from build123d import *

# Parameters (mm, degrees)
BOSS_EXTRU_1_DEPTH                                = 53.6
BOSS_EXTRU_1_DEPTH_BACK                           = 0.0001
ESQUISSE1_W                                       = 102.6
ESQUISSE1_H                                       = 35
ESQUISSE4_W                                       = 98.6
ESQUISSE4_H                                       = 51.6
ENL_V_MAT_EXTRU_2_DEPTH                           = 33
ESQUISSE9_W                                       = 10
ESQUISSE9_H                                       = 12.38
BOSS_EXTRU_3_DEPTH                                = 21.5
CONG_1_R                                          = 5
ESQUISSE10_R                                      = 3.75
ENL_V_MAT_EXTRU_4_DEPTH                           = 15
ENL_V_MAT_EXTRU_5_DEPTH                           = 2.1
ESQUISSE19_W                                      = 102.6
ESQUISSE19_H                                      = 53.6001
BOSS_EXTRU_4_DEPTH                                = 5
ESQUISSE21_W                                      = 5
ESQUISSE21_H                                      = 40
BOSS_EXTRU_5_DEPTH                                = 12
ESQUISSE22_W                                      = 5
ESQUISSE22_H                                      = 40
BOSS_EXTRU_6_DEPTH                                = 12
FRAISAGE_POUR_VIS_T_TE_FRAIS_E_BOMB_E_D           = 5.09999996
FRAISAGE_POUR_VIS_T_TE_FRAIS_E_BOMB_E_CSINK_D     = 10.500000082
FRAISAGE_POUR_VIS_T_TE_FRAIS_E_BOMB_E_CSINK_ANGLE = 90


with BuildPart() as part:
    # Esquisse1 → Boss.-Extru.1 (new, two sides: drawn at the far end of the back side and taken through both)
    with BuildSketch(Plane.XY.offset(-BOSS_EXTRU_1_DEPTH_BACK)):
        with Locations((33.832170394, 1.686746988)):
            Rectangle(ESQUISSE1_W, ESQUISSE1_H)
    extrude(amount=BOSS_EXTRU_1_DEPTH + BOSS_EXTRU_1_DEPTH_BACK)

    # Esquisse4 → Enlèv. mat.-Extru.2 (cut)
    with BuildSketch(Plane(origin=(0, 19.186746988, 0), x_dir=(1, 0, 0), z_dir=(0, 1, 0))):
        with Locations((33.832170394, -25.7999)):
            Rectangle(ESQUISSE4_W, ESQUISSE4_H)
    extrude(amount=-ENL_V_MAT_EXTRU_2_DEPTH, mode=Mode.SUBTRACT)

    # Esquisse9 → Boss.-Extru.3 (add)
    with BuildSketch(Plane(origin=(0, -13.813253012, 0), x_dir=(1, 0, 0), z_dir=(0, 1, 0))):
        with Locations((1.532170394, -32.0399)):
            Rectangle(ESQUISSE9_W, ESQUISSE9_H)
        with Locations((66.132170394, -32.0399)):
            Rectangle(ESQUISSE9_W, ESQUISSE9_H)
    extrude(amount=BOSS_EXTRU_3_DEPTH)

    # Congé1
    cong_1_edges = [part.edges().sort_by_distance(p)[0] for p in [
        (-3.467829606, 7.686746988, 32.0399),
        (6.532170394, 7.686746988, 32.0399),
        (71.132170394, 7.686746988, 32.0399),
        (61.132170394, 7.686746988, 32.0399),
    ]]
    fillet(cong_1_edges, radius=CONG_1_R - 0.0001)  # a hair under: the kernel refuses the full size

    # Esquisse10 → Enlèv. mat.-Extru.4 (cut)
    with BuildSketch(Plane(origin=(0, 0, 25.8499), x_dir=(-1, 0, 0), z_dir=(0, 0, -1))):
        with Locations((-66.132170394, 2.186746988)):
            Circle(ESQUISSE10_R)
        with Locations((-1.532170394, 2.186746988)):
            Circle(ESQUISSE10_R)
    extrude(amount=-ENL_V_MAT_EXTRU_4_DEPTH, mode=Mode.SUBTRACT)

    # Esquisse18 → Enlèv. mat.-Extru.5 (cut)
    with BuildSketch(Plane.XY.offset(53.6)):
        with BuildLine():
            Line((24.333519225, -13.813253012), (44.330821563, -13.813253012))
            ThreePointArc((44.330821563, -13.813253012), (34.332170394, -3.643205178), (24.333519225, -13.813253012))
        make_face()
    extrude(amount=-ENL_V_MAT_EXTRU_5_DEPTH, mode=Mode.SUBTRACT)

    # Esquisse19 → Boss.-Extru.4 (add)
    with BuildSketch(Plane.XZ.offset(15.813253012)):
        with Locations((33.832170394, 26.79995)):
            Rectangle(ESQUISSE19_W, ESQUISSE19_H)
    extrude(amount=BOSS_EXTRU_4_DEPTH)

    # Esquisse21 → Boss.-Extru.5 (add)
    with BuildSketch(Plane.ZY.offset(17.467829606)):
        with Locations((2.4999, -0.813253012)):
            Rectangle(ESQUISSE21_W, ESQUISSE21_H)
    extrude(amount=BOSS_EXTRU_5_DEPTH)

    # Esquisse22 → Boss.-Extru.6 (add)
    with BuildSketch(Plane(origin=(85.132170394, 0, 0), x_dir=(0, 0, -1), z_dir=(1, 0, 0))):
        with Locations((-2.4999, -0.813253012)):
            Rectangle(ESQUISSE22_W, ESQUISSE22_H)
    extrude(amount=BOSS_EXTRU_6_DEPTH)

    # Fraisage pour vis à tête fraisée bombée #51 (through all)
    with Locations(Plane(origin=(91.132170394, 13.186746988, -0.0001), x_dir=(-1, 0, 0), z_dir=(0, 0, -1))):
        with Locations((0, 0), (0, -28), (114.6, 0), (114.6, -28)):
            CounterSinkHole(FRAISAGE_POUR_VIS_T_TE_FRAIS_E_BOMB_E_D / 2, FRAISAGE_POUR_VIS_T_TE_FRAIS_E_BOMB_E_CSINK_D / 2, counter_sink_angle=FRAISAGE_POUR_VIS_T_TE_FRAIS_E_BOMB_E_CSINK_ANGLE)


solid = part.part
For this review, take the finished solid that the model builds, in its own axes (mm). A direction names the side the tool comes from. Give positions to 0.01 mm unless a question says otherwise; leave off trailing zeros. Loops run counter-clockwise (first coordinate to the right, second up) from the corner with the lowest first, then second, coordinate; pieces in that order, holes last. Notation, with made-up numbers: M 31,42.5 L 71,42.5 A32 cw 71,76.5 Z; hole C 30,32.5 d2. An arc over 180 degrees is marked long. Answer as a JSON object with one key per item and string values. Group by question number.
Q1. Add section B-B on x = 41. Give the boundary of the cut face in (y, z), and give its area (3 significant figures).
Q2. Mouldability with a two-part tool opening along Y and no side actions: class faces 1 (the conical face through (-20.91, 13.99, 2.57)), 2 (the flat face through (34, -14, 0)), 3 (the cylindrical face through (69.71, 6.18, 31.95)) as +Y half, -Y half, draft (parallel to the pull), parting line (faces both ways), or undercut.
Q3. For probe 1 along X at (y, z) = (1, 45.5); probe 2 along X at (y, z) = (-9, 28); probe 3 along X at (y, z) = (0, 27), list the stretches that pass through material, from the lowest coordinate up. Write a range as [from, to].
Q4. Add section A-A on z = 48. Give the boundary of the cut face in (x, y), and give its area (3 significant figures).
Q5. Insertion check: P1, Ø1.5, axis at x = 30.5, z = 40, coming from the +Y side; P2, Ø10, axis at y = -6, z = 29, coming from the -X side; P3, Ø6, axis at x = -23.5, y = -4.5, coming from the +Z side. Each pin has a flat end and moves straight along its axis. Give the tip position at first contact, or say it passes through.
Q6. Add section C-C on y = -5. Give the boundary of the cut face in (x, z), and give its area (3 significant figures).
Q7. Add section D-D on x = -11. Give the boundary of the cut face in (y, z).
Q8. Tool access review of faces 4 (the flat face through (85.132, -1, 29)), 5 (the flat face through (6.532, -6, 32)), 6 (the cylindrical face through (2.345, -1.474, 31.953)), 7 (the flat face through (97.132, -1, 3)), 8 (the flat face through (66, -6, 38.23)): name each direction out of +Z, -Z, +X, -X, +Y, -Y from which nothing blocks a thin tool from reaching the whole face with its end or side.
Checked values:
{
 "1": {"outline": "M -20.81,0 L -13.81,0 L -13.81,53.6 L -20.81,53.6 Z; M -6.19,51.6 L 19.19,51.6 L 19.19,53.6 L -6.19,53.6 Z", "area": "426 mm²"},
 "2": {"face 1": "undercut", "face 2": "draft", "face 3": "+Y half"},
 "3": {"probe 1": "[-17.47, -15.47], [83.13, 85.13]", "probe 2": "[-17.47, -15.47], [-3.47, 6.53], [61.13, 71.13], [83.13, 85.13]", "probe 3": "[-17.47, -15.47], [-3.47, -1.51], [4.58, 6.53], [61.13, 63.09], [69.18, 71.13], [83.13, 85.13]"},
 "4": {"outline": "M -17.47,-20.81 L 85.13,-20.81 L 85.13,19.19 L 83.13,19.19 L 83.13,-13.81 L -15.47,-13.81 L -15.47,19.19 L -17.47,19.19 Z", "area": "850 mm²"},
 "5": {"P1": "y = -13.81", "P2": "x = -17.47", "P3": "z = 5"},
 "6": {"outline": "M -29.47,0 L -15.47,0 L -15.47,51.6 L 29.3,51.6 L 29.3,53.6 L -17.47,53.6 L -17.47,5 L -29.47,5 Z; M -3.47,25.85 L 6.53,25.85 L 6.53,38.23 L -3.47,38.23 Z; M 39.36,51.6 L 83.13,51.6 L 83.13,0 L 97.13,0 L 97.13,5 L 85.13,5 L 85.13,53.6 L 39.36,53.6 Z; M 61.13,25.85 L 71.13,25.85 L 71.13,38.23 L 61.13,38.23 Z", "area": "759 mm²"},
 "7": {"outline": "M -20.81,0 L -13.81,0 L -13.81,51.6 L 19.19,51.6 L 19.19,53.6 L -20.81,53.6 Z"},
 "8": {"face 4": "+Z, +X, +Y, -Y", "face 5": "-Z, +Y", "face 6": "-Z", "face 7": "+Z, -Z, +X, +Y, -Y", "face 8": "+Y"}
}
